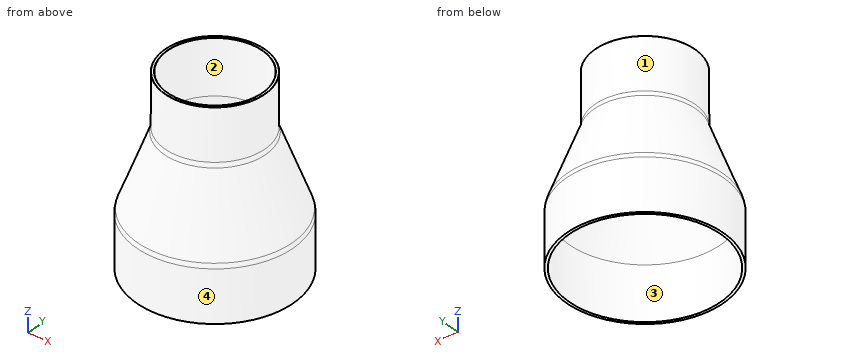
from build123d import *

# Parameters (mm, degrees)
F2_R = 5
F3_R = 0.1


with BuildPart() as f1:
    # F0 (on Front) → F1 (revolve)
    with BuildSketch(Plane.XZ):
        Polygon((-29, 20), (-29, 0), (-28, 0), (-28, 19.8192848565), (-17.5, 47.9217758492), (-17.5, 68.1024909928), (-18.5, 68.1024909928), (-18.5, 48.1024909928), align=None)
    revolve(axis=Axis((0, 0, 23.4480407089), (0, 0, 1)))

    # F2
    f2_edges = [f1.edges().sort_by_distance(p)[0] for p in [
        (29, 0, 20),
        (18.5, 0, 48.102491),
    ]]
    fillet(f2_edges, radius=F2_R)

    # F3
    f3_edges = [f1.edges().sort_by_distance(p)[0] for p in [
        (17.5, 0, 68.102491),
        (18.5, 0, 68.102491),
    ]]
    fillet(f3_edges, radius=F3_R)


solid = f1.part
Read the model definition and answer for the solid it produces. Units are mm, in the model's axes. Face numbers are marked on the shaded views. A direction names the side the tool comes from. Round coordinates to 2 decimals unless told otherwise and drop trailing zeros. Write each loop counter-clockwise with the first axis right and the second up, starting at its lowest first coordinate (ties: lowest second). Pieces come first, ordered by that corner, then holes.
Q1. A tool of negligible diameter and unlimited length cuts with its end or side. For the marked faces 3 and 4, from which of +Z, -Z, +X, -X, +Y, -Y can it reach the whole face along a straight path? Write none if from no direction.
Values:
face 3: -Z
face 4: +Z, -Z
Q2. Find section B-B on z = 33. Determine the outline of the cut face in (x, y).
Values:
outline: circle Ø48.29 at (0, 0); hole circle Ø46.15 at (0, 0)
Q3. Flat-ended cylindrical pins translate along their axes: P1, Ø2, axis at y = 5.5, z = 39, coming from the -X side; P2, Ø12, axis at x = -4.5, z = 13.5, coming from the -Y side; P3, Ø1.5, axis at y = -14.5, z = 13, coming from the +X side; P4, Ø6, axis at x = 11, z = 60.5, coming from the -Y side. Find the tip coordinate at first contact, or state that the pin passes through.
Values:
P1: stops at x = -21.65
P2: stops at y = -29
P3: stops at x = 25.53
P4: stops at y = -16.68
Q4. Find section A-A on z = 16.5. Determine the outline of the cut face in (x, y), and give its area (3 significant figures).
Values:
outline: circle Ø58 at (0, 0); hole circle Ø56 at (0, 0)
area: 179 mm2
Q5. Straight lines are drawn through the part: line 1 (Y direction, x = 0, z = 61.5); line 2 (X direction, y = 0, z = 13.25). For each, find the intervals that lie inside material, in ascending order.
Values:
line 1: y = -18.5 to -17.5, 17.5 to 18.5
line 2: x = -29 to -28, 28 to 29
Q6. The mould has two halves that part along Y. Classify the marked faces 1 and 2: released by +Y, released by -Y, zero draft, split by the parting line, or undercut.
Values:
face 1: split by the parting line
face 2: undercut
